The listing builds one solid part. Answer for the finished solid, in the listing's coordinates (mm). A direction names the side the tool comes from. Give positions to 0.01 mm unless a question says otherwise; leave off trailing zeros. Write each loop counter-clockwise with the first axis right and the second up, starting at its lowest first coordinate (ties: lowest second). Pieces come first, ordered by that corner, then holes. Notation, with made-up numbers: (66.25, 37) - (104.25, 37) arc R30 ccw to (104.25, 59) - close; hole circle Ø10 at (65, 44.25). An arc over 180 degrees is marked (long way). Return JSON: item names as keys, results as strings.
Autodesk Inventor part; units mm, degrees
ref_plane "YZ Plane" through (0, 0, 0) normal (1, 0, 0) x (0, 1, 0)
ref_plane "XZ Plane" through (0, 0, 0) normal (0, 1, 0) x (-1, 0, 0)
ref_plane "XY Plane" through (0, 0, 0) normal (0, 0, 1) x (1, 0, 0)
sketch "Эскиз1" plane through (0, 0, 0) normal (0, 0, 1) x (1, 0, 0)
  line L0 (33.5, -8.5) -> (33.5, 11.5)
  line L1 (28.5, 11.5) -> (-21.5, 11.5)
  line L2 (-21.5, 11.5) -> (-21.5, -8.5)
  line L3 (-21.5, -8.5) -> (28.5, -8.5)
  line L4 (28.5, -8.5) -> (28.5, 11.5)
  point P0 (0, 0)
  point P1 (28.5, 1.5)
  point P2 (33.5, 1.5)
  dimension "d0" = 20
  dimension "d1" = 50
  dimension "d2" = 5
extrude "Выдавливание1" add sketch "Эскиз1" along normal blind 35
sketch "Эскиз2" plane through (-21.5, 11.5, 0) normal (0, 1, 0) x (1, 0, 0)
  line L0 (34.9155, -7.2898) -> (19.9439, -7.2898)
  arc A0 (29.433, -14.5026) -> (34.9155, -7.2898) centre (27.4297, -7.2898) ccw
  line L1 (29.0336, -16.2113) -> (32.723, -19.5135)
  line L2 (32.723, -19.5135) -> (45.8164, -23.3718)
  line L3 (45.8164, -23.3718) -> (45.6044, -24.0912)
  line L4 (45.6044, -24.0912) -> (46.806, -24.4452)
  line L5 (46.806, -24.4452) -> (46.382, -25.8841)
  line L6 (46.382, -25.8841) -> (45.1805, -25.53)
  line L7 (45.1805, -25.53) -> (44.9685, -26.2494)
  line L8 (44.9685, -26.2494) -> (31.875, -22.3912)
  line L9 (31.875, -22.3912) -> (21.5, -16.6598)
  line L10 (21.5, -16.6598) -> (19.9439, -14.1649)
  line L11 (19.9439, -14.1649) -> (19.9439, -7.2898)
  line L12 (31.8727, -7.2898) -> (27.4716, -4.0907)
  line L13 (26.6475, -2.4729) -> (26.6475, 0)
  line L14 (0, 0) -> (50, 0)
  line L15 (12.3278, 0) -> (12.3278, -7.1542)
  line L16 (12.3278, -7.1542) -> (13.5221, -11.5576)
  line L17 (14.4853, -12.7847) -> (21.5, -16.6598)
  arc A1 (29.433, -14.5026) -> (29.0336, -16.2113) centre (29.7006, -15.4662) ccw
  arc A2 (13.5221, -11.5576) -> (14.4853, -12.7847) centre (15.4524, -11.0341) ccw
  arc A3 (26.6475, -2.4729) -> (27.4716, -4.0907) centre (28.6475, -2.4729) ccw
  point P0 (21.5, 0)
  point P1 (27.4297, -14.7757)
  point P2 (13.7439, -12.3751)
  dimension "d5" = 1
  dimension "d6" = 2
  dimension "d7" = 0.75
  dimension "d8" = 3
  dimension "d9" = 1.5
extrude "Выдавливание2" cut sketch "Эскиз2" against normal through all keep common part
sketch "Эскиз3" plane through (-9.1722, 11.5, 0) normal (-1, 0, 0) x (0, 0, 1)
  line L0 (26.2494, 0) -> (26.2494, -20)
  line L1 (12.7847, 0) -> (12.7847, -20)
  line L2 (26.2494, -7.5889) -> (12.7847, -7.5889)
  line L3 (12.7847, -7.5889) -> (12.7847, -12.5875)
  line L4 (12.7847, -12.5875) -> (26.2494, -12.5875)
  line L5 (26.2494, -12.5875) -> (26.2494, -7.5889)
  line L6 (7.2898, 0) -> (7.2898, -20)
  line L7 (12.7847, -3.5953) -> (7.2898, -3.5953)
  line L8 (7.2898, -3.5953) -> (7.2898, -16.3417)
  line L9 (7.2898, -16.3417) -> (12.7847, -16.3417)
  line L10 (12.7847, -16.3417) -> (12.7847, -3.5953)
  line L11 (0, -20) -> (0, 0)
  line L12 (7.2898, -5.3948) -> (0, -5.3948)
  line L13 (0, -5.3948) -> (0, -14.7921)
  line L14 (0, -14.7921) -> (7.2898, -14.7921)
  line L15 (7.2898, -14.7921) -> (7.2898, -5.3948)
  point P0 (0, -11.5)
  point P1 (12.7847, -7.5889)
  point P2 (7.2898, -3.5953)
  point P3 (7.2898, -5.3948)
  point P4 (0, -5.3948)
extrude "Выдавливание3" cut sketch "Эскиз3" against normal blind 35 keep common part
Item 1: The mould has two halves that part along Z. Classify faces 6 (the face through (9, 3.911, 19)), 7 (the face through (9.352, 1.447, 17.839)), 8 (the face through (7.23, 1.45, 15.22)), 9 (the face through (-8.583, 1.621, 9.325)): +Z half, -Z half, draft (parallel to the pull), parting line (faces both ways), or undercut.
Answer below:
{"face 6": "draft", "face 7": "undercut", "face 8": "undercut", "face 9": "+Z half"}
Item 2: A cutting plane is placed at C-C on z = 3. Determine the outline of the cut face in (x, y), then the cut area to 3 significant figures.
Answer below:
{"outline": "(-9.17, -3.29) - (5.22, -3.29) - (5.22, 6.11) - (-9.17, 6.11) - close", "area": "135 mm²"}
Item 3: For faces 1 (the face through (4.7, 6.3, 7.29)), 2 (the face through (9, -1.088, 19)), 3 (the face through (2, 6, 12.785)), 4 (the face through (24.697, 1.447, 24.266)), 5 (the face through (5.148, 1, 1)), determine the directions among +Z, -Z, +X, -X, +Y, -Y from which every point of the face is accessible in a straight line to the end or side of a thin tool.
Answer below:
{"face 1": "-Z, +X", "face 2": "+Z, +X, -X, -Y", "face 3": "+Z, +X, -X, +Y", "face 4": "+X, +Y, -Y", "face 5": "-Z, +X, +Y, -Y"}
Item 4: Consider L1, parallel to Z at x = 3, y = 6; L2, parallel to Y at x = 5, z = 16; L3, parallel to Z at x = -5, y = 6.75. Determine where each line is inside the solid, lowest interval first.
Answer below:
{"L1": "z = 0 to 12.78", "L2": "y = -1.09 to 3.91", "L3": "z = 7.29 to 12.78"}
Item 5: A cutting plane is placed at B-B on y = 0.5. Determine the outline of the cut face in (x, z) (1 decimal).
Answer below:
{"outline": "(-9.2, 0) - (5.1, 0) - (5.1, 2.5) arc R2 cw to (6, 4.1) - (10.4, 7.3) - (13.4, 7.3) arc R7.5 ccw to (7.9, 14.5) arc R1 cw to (7.5, 16.2) - (11.2, 19.5) - (24.3, 23.4) - (24.1, 24.1) - (25.3, 24.4) - (24.9, 25.9) - (23.7, 25.5) - (23.5, 26.2) - (10.4, 22.4) - (0, 16.7) - (-7, 12.8) arc R2 ccw to (-8, 11.6) - (-9.2, 7.2) - close"}
Item 6: A cutting plane is placed at D-D on x = 15. Determine the outline of the cut face in (y, z).
Answer below:
{"outline": "(-1.09, 20.63) - (3.91, 20.63) - (3.91, 23.75) - (-1.09, 23.75) - close"}
Item 7: Flat-ended cylindrical pins translate along their axes: P1, Ø6.5, axis at x = 9, z = 20.5, coming from the -Y side; P2, Ø2, axis at x = -1, z = 3, coming from the -Y side; P3, Ø2, axis at x = -3, z = 3.5, coming from the +Y side; P4, Ø5, axis at y = 6.5, z = 19, coming from the +X side. Find the tip coordinate at first contact, or state that the pin passes through.
Answer below:
{"P1": "stops at y = -1.09", "P2": "stops at y = -3.29", "P3": "stops at y = 6.11", "P4": "passes through"}
Item 8: A cutting plane is placed at A-A on y = -1.5. Determine the outline of the cut face in (x, z), then the cut area to 3 significant figures.
Answer below:
{"outline": "(-9.17, 0) - (5.15, 0) - (5.15, 2.47) arc R2 cw to (5.97, 4.09) - (10.37, 7.29) - (13.42, 7.29) arc R7.49 ccw to (11.01, 12.78) - (-7.01, 12.78) arc R2 ccw to (-7.98, 11.56) - (-9.17, 7.15) - close", "area": "230 mm²"}
